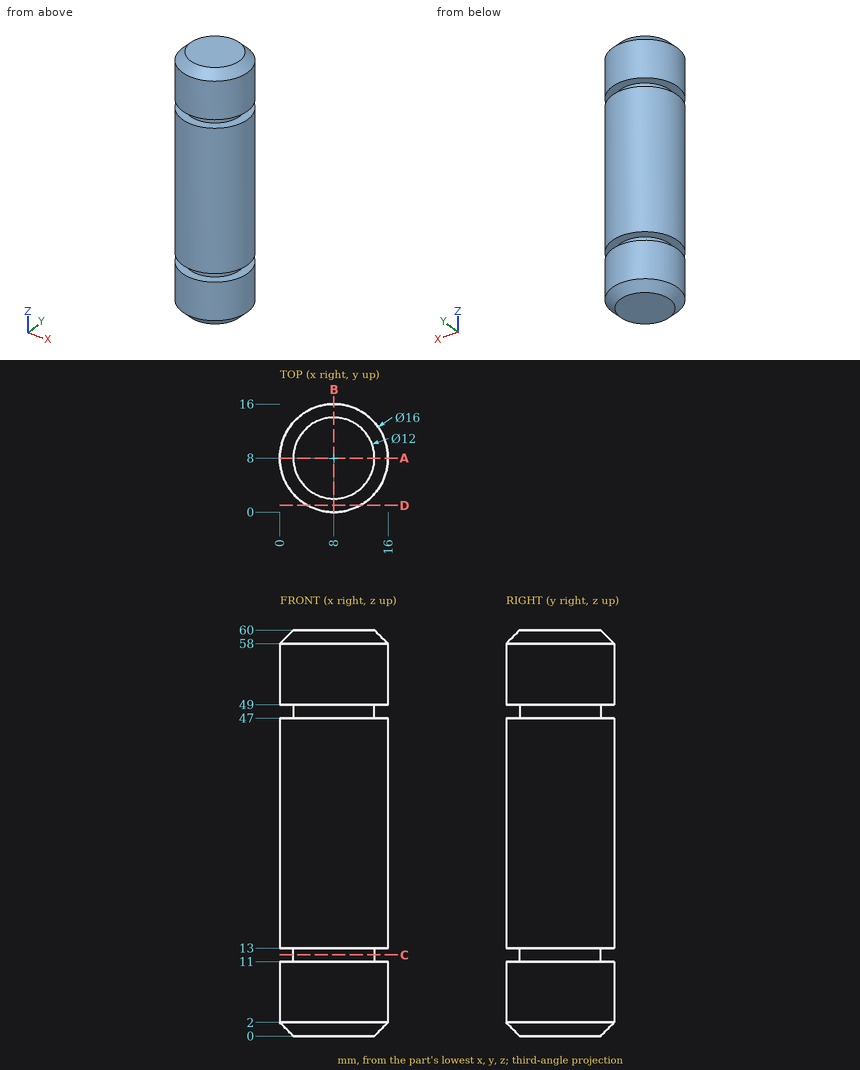
Geometry check sheet. Reference: drawing and pictorial views, mm from the part's lowest x, y, z. Give positions to 0.01 mm unless a question says otherwise; leave off trailing zeros. Loops run counter-clockwise (first coordinate to the right, second up) from the corner with the lowest first, then second, coordinate; pieces in that order, holes last. Notation, with made-up numbers: M 71.5,72 L 127.5,72 A11 ccw 127.5,82 Z; hole C -10,63 d5. An arc over 180 degrees is marked long. One line per question, with ' | ' between items.
Item 1: Depth check by flat-ended pin: P1, Ø1, axis at x = 13, y = 14, coming from the -Z side; P2, Ø1, axis at y = 3, z = 42.5, coming from the -X side; P3, Ø1, axis at y = 2.5, z = 43.5, coming from the -X side (3 decimals). Enter the tip coordinate at first touch or a pass-through.
Completed:
P1: stops at z = 1.31 | P2: stops at x = 1.39 | P3: stops at x = 1.755
Item 2: Section check C-C, the plane z = 12. Record the cut outline in (x, y).
Completed:
outline: C 8,8 d12
Item 3: Thickness scan on line 1 (Z direction, x = 9, y = 1); line 2 (Z direction, x = 4.75, y = 2); line 3 (X direction, y = 8.25, z = 37.5). Record the ranges inside material, lowest first. Write a range as [from, to].
Completed:
line 1: z = [1.07, 11], [13, 47], [49, 58.93] | line 2: z = [0.82, 11], [13, 47], [49, 59.18] | line 3: x = [0, 16]
Item 4: Section check D-D, the plane y = 1. State how many separate pieces and enclosed holes the cut face has, plus the area to 3 significant figures.
Completed:
separate pieces: 3 | enclosed holes: 0 | area: 413 mm^2
Item 5: Section check A-A, the plane y = 8. Record the cut outline in (x, z), plus the area to 3 significant figures.
Completed:
outline: M 0,2 L 2,0 L 14,0 L 16,2 L 16,11 L 14,11 L 14,13 L 16,13 L 16,47 L 14,47 L 14,49 L 16,49 L 16,58 L 14,60 L 2,60 L 0,58 L 0,49 L 2,49 L 2,47 L 0,47 L 0,13 L 2,13 L 2,11 L 0,11 Z | area: 936 mm^2
